```python
from build123d import *

# Parameters (mm, degrees)
ESQUISSE1_R        = 1.75
BOSS_EXTRU_1_DEPTH = 40


with BuildPart() as part:
    # Esquisse1 → Boss.-Extru.1 (new body)
    with BuildSketch(Plane.XY):
        with BuildLine():
            Line((-1.5, 5), (-5, 5))
            Line((-5, 5), (-5, 1.5))
            Line((-5, 1.5), (-4, 1.5))
            Line((-4, 1.5), (-4, 2.5))
            Line((-4, 2.5), (-3.207106781, 2.5))
            Line((-3.207106781, 2.5), (-2.216672281, 1.15601211))
            ThreePointArc((-2.216672281, 1.15601211), (-2.5, 0), (-2.216672281, -1.15601211))
            Line((-2.216672281, -1.15601211), (-3.207106781, -2.5))
            Line((-3.207106781, -2.5), (-4, -2.5))
            Line((-4, -2.5), (-4, -1.5))
            Line((-4, -1.5), (-5, -1.5))
            Line((-5, -1.5), (-5, -5))
            Line((-5, -5), (-1.5, -5))
            Line((-1.5, -5), (-1.5, -4))
            Line((-1.5, -4), (-2.5, -4))
            Line((-2.5, -4), (-2.5, -3.207106781))
            Line((-2.5, -3.207106781), (-1.15601211, -2.216672281))
            ThreePointArc((-1.15601211, -2.216672281), (0, -2.5), (1.15601211, -2.216672281))
            Line((1.15601211, -2.216672281), (2.5, -3.207106781))
            Line((2.5, -3.207106781), (2.5, -4))
            Line((2.5, -4), (1.5, -4))
            Line((1.5, -4), (1.5, -5))
            Line((1.5, -5), (5, -5))
            Line((5, -5), (5, -1.5))
            Line((5, -1.5), (4, -1.5))
            Line((4, -1.5), (4, -2.5))
            Line((4, -2.5), (3.207106781, -2.5))
            Line((3.207106781, -2.5), (2.216672281, -1.15601211))
            ThreePointArc((2.216672281, -1.15601211), (2.5, 0), (2.216672281, 1.15601211))
            Line((2.216672281, 1.15601211), (3.207106781, 2.5))
            Line((3.207106781, 2.5), (4, 2.5))
            Line((4, 2.5), (4, 1.5))
            Line((4, 1.5), (5, 1.5))
            Line((5, 1.5), (5, 5))
            Line((5, 5), (1.5, 5))
            Line((1.5, 5), (1.5, 4))
            Line((1.5, 4), (2.5, 4))
            Line((2.5, 4), (2.5, 3.207106781))
            Line((2.5, 3.207106781), (1.15601211, 2.216672281))
            ThreePointArc((1.15601211, 2.216672281), (0, 2.5), (-1.15601211, 2.216672281))
            Line((-1.15601211, 2.216672281), (-2.5, 3.207106781))
            Line((-2.5, 3.207106781), (-2.5, 4))
            Line((-2.5, 4), (-1.5, 4))
            Line((-1.5, 4), (-1.5, 5))
        make_face()
        Polygon((-4.75, 1.75), (-4.75, 4.75), (-1.75, 4.75), (-1.75, 4.25), (-2.75, 4.25), (-2.75, 2.75), (-4.25, 2.75), (-4.25, 1.75), align=None, mode=Mode.SUBTRACT)
        Circle(ESQUISSE1_R, mode=Mode.SUBTRACT)
        Polygon((-4.75, -4.75), (-4.75, -1.75), (-4.25, -1.75), (-4.25, -2.75), (-2.75, -2.75), (-2.75, -4.25), (-1.75, -4.25), (-1.75, -4.75), align=None, mode=Mode.SUBTRACT)
        Polygon((4.75, 4.75), (4.75, 1.75), (4.25, 1.75), (4.25, 2.75), (2.75, 2.75), (2.75, 4.25), (1.75, 4.25), (1.75, 4.75), align=None, mode=Mode.SUBTRACT)
        Polygon((4.75, -4.75), (1.75, -4.75), (1.75, -4.25), (2.75, -4.25), (2.75, -2.75), (4.25, -2.75), (4.25, -1.75), (4.75, -1.75), align=None, mode=Mode.SUBTRACT)
    extrude(amount=BOSS_EXTRU_1_DEPTH)


solid = part.part
```
Could you check a few things on this model? Use its own coordinates, in mm. A direction names the side the tool comes from. Give positions to 0.01 mm unless a question says otherwise; leave off trailing zeros. Loops run counter-clockwise (first coordinate to the right, second up) from the corner with the lowest first, then second, coordinate; pieces in that order, holes last. Notation, with made-up numbers: (56.5, 85) -> (99.5, 85) arc R16 cw to (99.5, 112) -> close; hole circle Ø2 at (-30.75, -36). An arc over 180 degrees is marked (long way). Put each result on its own line as item: value.
(1) Thinking about a two-plate mould opening in X: for faces 1 (the face through (-2.5, 0, 19.7)), 2 (the face through (4.5, 1.5, 19.7)), 3 (the face through (2, -4, 20)), which applies, pulls with the +X half, pulls with the -X half, needs draft (parallel to the pull), parting line crosses it, or undercut?
Computed:
face 1: pulls with the -X half
face 2: needs draft
face 3: undercut
(2) Imagine slicing it at C-C on z = 33.5. State how many separate pieces and enclosed holes the cut face has, plus the area to 3 significant figures.
Computed:
separate pieces: 1
enclosed holes: 5
area: 29.8 mm^2
(3) For faces 4 (the face through (1.5, 4.5, 19.7)), 5 (the face through (-5, -3, 20)), 6 (the face through (1.819, -2.705, 19.72)), which set-ups out of +Z, -Z, +X, -X, +Y, -Y let a thin tool reach every point of the face, with its end or its side?
Computed:
face 4: +Z, -Z, +Y
face 5: +Z, -Z, -X, +Y, -Y
face 6: +Z, -Z
(4) Please list where these lines run through material, in increasing order: probe 1 along X at (y, z) = (-3.25, 14.5); probe 2 along Y at (x, z) = (0, 11.5). Write a range as [from, to].
Computed:
probe 1: [-5, -4.75], [-2.75, -2.5], [2.5, 2.75], [4.75, 5]
probe 2: [-2.5, -1.75], [1.75, 2.5]
(5) Imagine slicing it at A-A on y = 0. Write out the boundary of the cut face in (x, z).
Computed:
outline: (-2.5, 0) -> (-1.75, 0) -> (-1.75, 40) -> (-2.5, 40) -> close; (1.75, 0) -> (2.5, 0) -> (2.5, 40) -> (1.75, 40) -> close
